from build123d import *

# Parameters (mm, degrees)
SKETCH1_R           = 1.5
SKETCH1_W           = 4
SKETCH1_H           = 1.5
BOSS_EXTRUDE1_DEPTH = 3


with BuildPart() as part:
    # Sketch1 → Boss-Extrude1 (new body)
    with BuildSketch(Plane(origin=(0, 0, 0), x_dir=(1, 0, 0), z_dir=(0, 1, 0))):
        Polygon((0, 129), (0, 169), (12, 169), (12, 129), (42, 129), (42, 0), (0, 0), align=None)
        with Locations(Location((19, 122.5, 0), (0, 0, 270))):
            Circle(SKETCH1_R, mode=Mode.SUBTRACT)
        with Locations(Location((35, 122.5, 0), (0, 0, 270))):
            Circle(SKETCH1_R, mode=Mode.SUBTRACT)
        with Locations((6, 164.75)):
            Rectangle(SKETCH1_W, SKETCH1_H, mode=Mode.SUBTRACT)
    extrude(amount=BOSS_EXTRUDE1_DEPTH)


solid = part.part
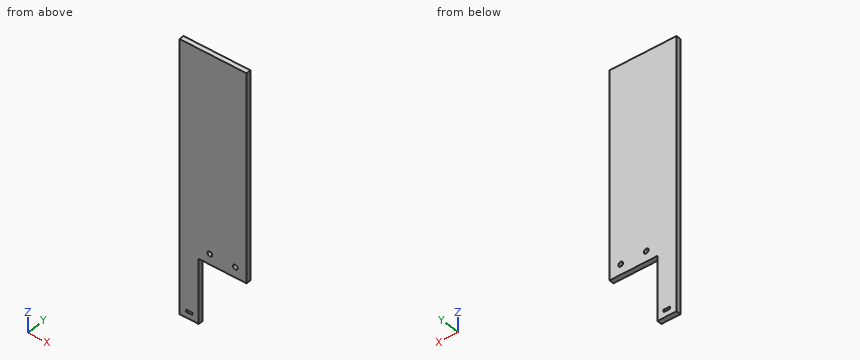
Geometry: final body of the model. Coordinates: model frame, mm. Coordinates: 2 decimals unless noted, no trailing zeros. Loops run counter-clockwise (first coordinate to the right, second up) from the corner with the lowest first, then second, coordinate; pieces in that order, holes last. Notation, with made-up numbers: (66, 15) - (105, 15) arc R15 cw to (105, 35) - close; hole circle Ø5 at (64, 47). An arc over 180 degrees is marked (long way). Put each result on its own line as item: value. Start each with the question number.
Q1. Cut plane B-B, the plane y = 2.5. Return loops of the section in (x, z), and give its area (3 significant figures).
Q2. Line query: line 1 (X direction, y = 0.95, z = -122.5); line 2 (Z direction, x = 33, y = 0.5); line 3 (Z direction, x = 20, y = 2.25). Output: solid intervals per line, ascending.
Q3. Pin query (flat end, axial travel): pin 1 Ø0.9 at (y, z) = (1.5, -148) entering from +X; pin 2 Ø1.5 at (x, y) = (33, 2) entering from -Z. Return the tip coordinate at first contact, or that it passes through.
Q4. Cut plane C-C, the plane x = 19. Return loops of the section in (y, z), and give its area (3 significant figures).
Q5. Cut plane D-D, the plane z = -156. Return loops of the section in (x, y), and give its area (3 significant figures).
Q6. Cut plane A-A, the plane z = -122.5. Return loops of the section in (x, y), and give its area (3 significant figures).
Filled sheet:
1. outline: (0, -169) - (12, -169) - (12, -129) - (42, -129) - (42, 0) - (0, 0) - close; hole (4, -165.5) - (8, -165.5) - (8, -164) - (4, -164) - close; hole circle Ø3 at (19, -122.5); hole circle Ø3 at (35, -122.5)
1. area: 5,880 mm²
2. line 1: 0 to 17.5, 20.5 to 33.5, 36.5 to 42
2. line 2: -129 to 0
2. line 3: -129 to -123.62, -121.38 to 0
3. pin 1: x = 12
3. pin 2: z = -129
4. outline: (0, -129) - (3, -129) - (3, -124) - (0, -124) - close; (0, -121) - (3, -121) - (3, 0) - (0, 0) - close
4. area: 378 mm²
5. outline: (0, 0) - (12, 0) - (12, 3) - (0, 3) - close
5. area: 36.0 mm²
6. outline: (0, 0) - (17.5, 0) - (17.5, 3) - (0, 3) - close; (20.5, 0) - (33.5, 0) - (33.5, 3) - (20.5, 3) - close; (36.5, 0) - (42, 0) - (42, 3) - (36.5, 3) - close
6. area: 108 mm²
